from build123d import *

# Parameters (mm, degrees)
SKETCH_1_R          = 30
SKETCH_1_R_2        = 24
EXTRUDE_1_DEPTH     = 5
SKETCH_2_R          = 1
CUT_EXTRUDE_1_DEPTH = 43.720018727
EXTRUDE_START       = -5
EXTRUDE_2_DEPTH     = 5


with BuildPart() as part:
    # 草图1 → 凸台-拉伸1 (new body)
    with BuildSketch(Plane.XY):
        Circle(SKETCH_1_R)
        Circle(SKETCH_1_R_2, mode=Mode.SUBTRACT)
    extrude(amount=EXTRUDE_1_DEPTH)

    # 草图2 → 切除-拉伸1 (cut, through all)
    with BuildSketch(Plane.XY.offset(5)):
        with Locations((0, 27)):
            Circle(SKETCH_2_R)
        with Locations((23.382685902, 13.5)):
            Circle(SKETCH_2_R)
        with Locations((23.382685902, -13.5)):
            Circle(SKETCH_2_R)
        with Locations((0, -27)):
            Circle(SKETCH_2_R)
        with Locations((-23.382685902, -13.5)):
            Circle(SKETCH_2_R)
        with Locations((-23.382685902, 13.5)):
            Circle(SKETCH_2_R)
    extrude(amount=-CUT_EXTRUDE_1_DEPTH, mode=Mode.SUBTRACT)

    # 草图3 → 凸台-拉伸2 (add)
    with BuildSketch(Plane.XY.offset(5).offset(EXTRUDE_START)):
        with BuildLine():
            Line((5.435199947, 20.284442352), (6.211657082, 23.182219831))
            ThreePointArc((6.211657082, 23.182219831), (3.132628613, 23.794676673), (0, 24))
            Line((0, 24), (0, 21))
            ThreePointArc((0, 21), (2.741050037, 20.820342089), (5.435199947, 20.284442352))
        make_face()
        with BuildLine():
            Line((0, 30), (0, 33))
            ThreePointArc((0, 33), (-4.307364343, 32.717680425), (-8.541028488, 31.875552268))
            Line((-8.541028488, 31.875552268), (-7.764571353, 28.977774789))
            ThreePointArc((-7.764571353, 28.977774789), (-3.915785767, 29.743345841), (0, 30))
        make_face()
    extrude(amount=EXTRUDE_2_DEPTH)


solid = part.part
Could you check a few things on this model? Use its own coordinates, in mm. A direction names the side the tool comes from. Coordinates: 2 decimals unless noted, no trailing zeros. Order: outer loops, then holes, each group sorted by start corner. A loop starts at its lowest first (then second) coordinate and runs counter-clockwise, first axis right, second up. Notation, with made-up numbers: (76, 43.5) -> (108, 43.5) arc R18 cw to (108, 58.5) -> close; hole circle Ø10 at (28.5, 2.25). An arc over 180 degrees is marked (long way). One line per item, written item: value. Start each with the question number.
1) Imagine slicing it at A-A on y = 0. List the corners of the cut face in (x, z) for me, plus the area to 3 significant figures.
2) I'm going to push flat-ended pins straight in: pin 1 (3 mm diameter, centred on x = -13.5, z = 2, fed in from -Y); pin 2 (2.5 mm diameter, centred on y = 23, z = 3.5, fed in from -X); pin 3 (1 mm diameter, centred on x = -16.5, z = 0.5, fed in from -Y). Where does each tip first touch, or does it pass through?
3) If I drill on L1, parallel to X at y = -13, z = 3.45; L2, parallel to X at y = 22, z = 4.3; L3, parallel to X at y = 10.5, z = 2.45, over which ranges is the centre line in solid material (lowest first)? Write a range as [from, to].
4) Imagine slicing it at D-D on x = 26. List the corners of the cut face in (y, z) for me, plus the area to 3 significant figures.
5) Imagine slicing it at C-C on y = 13.5. List the corners of the cut face in (x, z) for me.
6) Which directions (+Z, -Z, +X, -X, +Y, -Y) give clear straight access to the entire face, cutting with the end or side of a thin tool? Please do faces 1 (the cylindrical face through (-4.247, 32.726, 2.465)), 2 (the flat face through (-8.16, 30.45, 2.46)), 3 (the flat face through (5.818, 21.713, 2.465)), 4 (the flat face through (0, 31, 2)).
7) Imagine slicing it at B-B on x = -14.5. List the corners of the cut face in (y, z) for me.
Answer list:
1. outline: (-30, 0) -> (-24, 0) -> (-24, 5) -> (-30, 5) -> close; (24, 0) -> (30, 0) -> (30, 5) -> (24, 5) -> close
1. area: 60.0 mm2
2. pin 1: stops at y = -27.5
2. pin 2: stops at x = -20.66
2. pin 3: stops at y = -25.38
3. L1: x = [-27.04, -24.25], [-22.52, -20.17], [20.17, 22.52], [24.25, 27.04]
3. L2: x = [-20.4, -9.59], [0, 5.89], [9.59, 20.4]
3. L3: x = [-28.1, -21.58], [21.58, 28.1]
4. outline: (-14.97, 0) -> (14.97, 0) -> (14.97, 5) -> (-14.97, 5) -> close
4. area: 150 mm2
5. outline: (-26.79, 0) -> (-24.38, 0) -> (-24.38, 5) -> (-26.79, 5) -> close; (-22.38, 0) -> (-19.84, 0) -> (-19.84, 5) -> (-22.38, 5) -> close; (19.84, 0) -> (22.38, 0) -> (22.38, 5) -> (19.84, 5) -> close; (24.38, 0) -> (26.79, 0) -> (26.79, 5) -> (24.38, 5) -> close
6. face 1: +Z, -Z, -X, +Y
6. face 2: +Z, -Z, -X
6. face 3: +Z, -Z
6. face 4: +Z, -Z, +X, +Y
7. outline: (-26.26, 0) -> (-19.12, 0) -> (-19.12, 5) -> (-26.26, 5) -> close; (19.12, 0) -> (26.26, 0) -> (26.26, 5) -> (19.12, 5) -> close
